Read the model definition and answer for the solid it produces. Units are mm, in the model's axes. Coordinates: 2 decimals unless noted, no trailing zeros. Write each loop counter-clockwise with the first axis right and the second up, starting at its lowest first coordinate (ties: lowest second). Pieces come first, ordered by that corner, then holes. Notation, with made-up numbers: (20, 22) -> (31, 22) arc R32 ccw to (31, 55) -> close; hole circle Ø6 at (84.5, -10.5). An arc over 180 degrees is marked (long way). Write item = value, one per line. Start each with the question number.
1) Find the intervals of material crossed by line 1 along Z through (x, y) = (52.5, 2.65); line 2 along X through (y, z) = (1.75, 0); line 3 along X through (y, z) = (3.75, 16.5), in increasing order. Write a range as from..to.
2) Section C-C (x = 52.5) is taken. Determine the outline of the cut face in (y, z).
3) Section A-A (z = -16.11) is taken. Count the separate pieces of the cut face and the enclosed holes in it, plus the area to 3 significant figures.
4) For a pull along X with two mould halves and no side action, classify faces 1 (the face through (-15.004, 4.105, 18.024)), 2 (the face through (70, 4, 0)), 3 (the face through (-1, 4, 25)) as released by +X, released by -X, zero draft, split by the parting line, or undercut.
5) Section D-D (z = -0.5) is taken. Determine the outline of the cut face in (x, y).
6) Section B-B (x = 35) is taken. Determine the outline of the cut face in (y, z).
7) Flat-ended cylindrical pins translate along their axes: pin 1 Ø16.5 at (x, z) = (0, 0) entering from +Y; pin 2 Ø9.5 at (x, z) = (-17.5, 16.11) entering from -Y; pin 3 Ø8 at (x, z) = (-52.5, 16.11) entering from +Y. Find the tip coordinate at first contact, or state that the pin passes through.
from build123d import *

# Parameters (mm, degrees)
SKETCH1_W                                         = 140
SKETCH1_H                                         = 50
BOSS_EXTRUDE2_DEPTH                               = 6.5
SKETCH2_R                                         = 10.25
CUT_EXTRUDE1_DEPTH                                = 12.7
LPATTERN1_COUNT                                   = 2
LPATTERN1_PITCH                                   = 35
LPATTERN1_COL_COUNT                               = 2
LPATTERN1_COL_PITCH                               = 35
CSK_FOR_6_FLAT_HEAD_MACHINE_SCREW_100_D           = 6
CSK_FOR_6_FLAT_HEAD_MACHINE_SCREW_100_CSINK_D     = 12
CSK_FOR_6_FLAT_HEAD_MACHINE_SCREW_100_CSINK_ANGLE = 100
LPATTERN2_COUNT                                   = 4
LPATTERN2_PITCH                                   = 35
LPATTERN2_COUNT_DIR2                              = 2
LPATTERN2_PITCH_DIR2                              = 32.2199
CHAMFER1_SIZE                                     = 1.27


with BuildPart() as part:
    # Sketch1 → Boss-Extrude2 (new body)
    with BuildSketch(Plane(origin=(0, 0, 0), x_dir=(1, 0, 0), z_dir=(0, 1, 0))):
        Rectangle(SKETCH1_W, SKETCH1_H)
    extrude(amount=BOSS_EXTRUDE2_DEPTH)

    # Sketch2 → Cut-Extrude1 (cut)
    with BuildSketch(Plane(origin=(0, 6.5, 0), x_dir=(1, 0, 0), z_dir=(0, 1, 0))):
        with Locations(Location((0, 0, 0), (0, 0, 270))):
            Circle(SKETCH2_R)
    cut_extrude1 = extrude(amount=-CUT_EXTRUDE1_DEPTH, mode=Mode.SUBTRACT)

    # LPattern1: Cut-Extrude1 ×2
    with Locations(*[(i * LPATTERN1_PITCH, 0, 0) for i in range(1, LPATTERN1_COUNT)]):
        add(cut_extrude1, mode=Mode.SUBTRACT)

    # LPattern1 col: Cut-Extrude1 ×2
    with Locations(*[(-i * LPATTERN1_COL_PITCH, 0, 0) for i in range(1, LPATTERN1_COL_COUNT)]):
        add(cut_extrude1, mode=Mode.SUBTRACT)

    # CSK for #6 Flat Head Machine Screw (100)1 (through all)
    with Locations(Plane(origin=(0, 6.5, 0), x_dir=(1, 0, 0), z_dir=(0, 1, 0))):
        with Locations((-52.5, 16.11)):
            csk_for_6_flat_head_machine_screw_100 = CounterSinkHole(CSK_FOR_6_FLAT_HEAD_MACHINE_SCREW_100_D / 2, CSK_FOR_6_FLAT_HEAD_MACHINE_SCREW_100_CSINK_D / 2, counter_sink_angle=CSK_FOR_6_FLAT_HEAD_MACHINE_SCREW_100_CSINK_ANGLE)

    # LPattern2: CSK for _6 Flat Head Machine Screw _100 4 × 2
    with Locations(*[(i * LPATTERN2_PITCH, 0, j * LPATTERN2_PITCH_DIR2) for i in range(LPATTERN2_COUNT) for j in range(LPATTERN2_COUNT_DIR2) if (i, j) != (0, 0)]):
        add(csk_for_6_flat_head_machine_screw_100, mode=Mode.SUBTRACT)

    # Chamfer1
    chamfer1_edges = [part.edges().sort_by_distance(p)[0] for p in [
        (0, 0, 25),
        (-70, 0, 0),
        (0, 0, -25),
        (70, 0, 0),
    ]]
    chamfer(chamfer1_edges, length=CHAMFER1_SIZE)


solid = part.part
Answer key:
q1.line_1 = -25..-19.11, -13.11..13.11, 19.11..25
q1.line_2 = -70..-45.25, -24.75..-10.25, 10.25..24.75, 45.25..70
q1.line_3 = -70..-55.47, -49.53..-20.47, -14.53..14.53, 20.47..49.53, 55.47..70
q2.outline = (0, -23.73) -> (1.27, -25) -> (6.5, -25) -> (6.5, -22.11) -> (3.98, -19.11) -> (0, -19.11) -> close; (0, -13.11) -> (3.98, -13.11) -> (6.5, -10.11) -> (6.5, 10.11) -> (3.98, 13.11) -> (0, 13.11) -> close; (0, 19.11) -> (3.98, 19.11) -> (6.5, 22.11) -> (6.5, 25) -> (1.27, 25) -> (0, 23.73) -> close
q3.separate_pieces = 5
q3.enclosed_holes = 0
q3.area = 722 mm^2
q4.face_1 = undercut
q4.face_2 = released by +X
q4.face_3 = zero draft
q5.outline = (-70, 1.27) -> (-68.73, 0) -> (-45.24, 0) -> (-45.24, 6.5) -> (-70, 6.5) -> close; (-24.76, 0) -> (-10.24, 0) -> (-10.24, 6.5) -> (-24.76, 6.5) -> close; (10.24, 0) -> (24.76, 0) -> (24.76, 6.5) -> (10.24, 6.5) -> close; (45.24, 0) -> (68.73, 0) -> (70, 1.27) -> (70, 6.5) -> (45.24, 6.5) -> close
q6.outline = (0, -23.73) -> (1.27, -25) -> (6.5, -25) -> (6.5, -10.25) -> (0, -10.25) -> close; (0, 10.25) -> (6.5, 10.25) -> (6.5, 25) -> (1.27, 25) -> (0, 23.73) -> close
q7.pin_1 = through
q7.pin_2 = 0
q7.pin_3 = 4.82
